For this review, take the finished solid that the model builds, in its own axes (mm). Face numbers are marked on the shaded views. A direction names the side the tool comes from. Coordinates: 2 decimals unless noted, no trailing zeros. Write each loop counter-clockwise with the first axis right and the second up, starting at its lowest first coordinate (ties: lowest second). Pieces come first, ordered by that corner, then holes.
```python
from build123d import *
from OCP.BRepFilletAPI import BRepFilletAPI_MakeChamfer

# Parameters (mm, degrees)
SKETCH1_W           = 96.449496644
SKETCH1_H           = 93.866027984
BOSS_EXTRUDE1_DEPTH = 50
DRAFT1_ANGLE        = 20
CHAMFER1_SIZE       = 5
CHAMFER1_SIZE2      = 8.365785926
CHAMFER2_SIZE       = 2
CHAMFER2_SIZE2      = 3.34631437
SHELL1_T            = -3


with BuildPart() as part:
    # Sketch1 → Boss-Extrude1 (new body)
    with BuildSketch(Plane(origin=(0, 0, 0), x_dir=(1, 0, 0), z_dir=(0, 1, 0))):
        Rectangle(SKETCH1_W, SKETCH1_H)
        Polygon((20.883038336, 70.399520989), (48.224748322, 46.933013992), (-48.224748322, 46.933013992), (-20.883038336, 70.399520989), align=None)
        Polygon((-48.224748322, -46.933013992), (48.224748322, -46.933013992), (20.883038336, -70.399520989), (-20.883038336, -70.399520989), align=None)
    extrude(amount=BOSS_EXTRUDE1_DEPTH)

    # Draft1
    draft1_faces = [part.faces().sort_by_distance(p)[0] for p in [
        (-34.553893329, 25, 58.66626749),
        (-48.224748322, 25, 0),
        (-34.553893329, 25, -58.66626749),
        (0, 25, -70.399520989),
        (34.553893329, 25, -58.66626749),
        (48.224748322, 25, 0),
        (34.553893329, 25, 58.66626749),
        (0, 25, 70.399520989),
    ]]
    draft(draft1_faces, Plane(origin=(0, 0, 0), x_dir=(0, 0, -1), z_dir=(0, -1, 0)), DRAFT1_ANGLE)

    # Chamfer1: one chamfer whose edges measure the first distance from different faces: ONE call of the kernel's chamfer builder (chamfer() names one face for all edges)
    chamfer1_edges_1 = [part.edges().sort_by_distance(p)[0] for p in [
        (0, 0, 70.399520989),
        (-34.553893329, 0, 58.66626749),
        (34.553893329, 0, 58.66626749),
    ]]
    chamfer1_side_1 = [part.faces().sort_by_distance(p)[0] for p in [
        (0, 0, 0),
    ]]
    chamfer1_edges_2 = [part.edges().sort_by_distance(p)[0] for p in [
        (-34.553893329, 0, -58.66626749),
    ]]
    chamfer1_side_2 = [part.faces().sort_by_distance(p)[0] for p in [
        (-41.148260159, 26.443805038, -65.690138569),
    ]]
    chamfer1_edges_3 = [part.edges().sort_by_distance(p)[0] for p in [
        (0, 0, -70.399520989),
    ]]
    chamfer1_side_3 = [part.faces().sort_by_distance(p)[0] for p in [
        (0, 26.157748942, -79.920162999),
    ]]
    chamfer1_edges_4 = [part.edges().sort_by_distance(p)[0] for p in [
        (34.553893329, 0, -58.66626749),
    ]]
    chamfer1_side_4 = [part.faces().sort_by_distance(p)[0] for p in [
        (41.148260159, 26.443805038, -65.690138569),
    ]]
    chamfer1 = BRepFilletAPI_MakeChamfer(part.part.solid().wrapped)
    for e in chamfer1_edges_1:
        chamfer1.Add(CHAMFER1_SIZE, CHAMFER1_SIZE2, e.wrapped, chamfer1_side_1[0].wrapped)  # the first distance lies on this face
    for e in chamfer1_edges_2:
        chamfer1.Add(CHAMFER1_SIZE, CHAMFER1_SIZE2, e.wrapped, chamfer1_side_2[0].wrapped)  # the first distance lies on this face
    for e in chamfer1_edges_3:
        chamfer1.Add(CHAMFER1_SIZE, CHAMFER1_SIZE2, e.wrapped, chamfer1_side_3[0].wrapped)  # the first distance lies on this face
    for e in chamfer1_edges_4:
        chamfer1.Add(CHAMFER1_SIZE, CHAMFER1_SIZE2, e.wrapped, chamfer1_side_4[0].wrapped)  # the first distance lies on this face
    add(Compound.cast(chamfer1.Shape()), mode=Mode.REPLACE)

    # Chamfer2: one chamfer whose edges measure the first distance from different faces: ONE call of the kernel's chamfer builder (chamfer() names one face for all edges)
    chamfer2_edges_1 = [part.edges().sort_by_distance(p)[0] for p in [
        (48.224748322, 0, 2.217733352),
    ]]
    chamfer2_side_1 = [part.faces().sort_by_distance(p)[0] for p in [
        (57.660024046, 25.923206996, -0.008470654),
    ]]
    chamfer2_edges_2 = [part.edges().sort_by_distance(p)[0] for p in [
        (-48.224748322, 0, 2.217733352),
    ]]
    chamfer2_side_2 = [part.faces().sort_by_distance(p)[0] for p in [
        (0, 0, 1.984639343),
    ]]
    chamfer2 = BRepFilletAPI_MakeChamfer(part.part.solid().wrapped)
    for e in chamfer2_edges_1:
        chamfer2.Add(CHAMFER2_SIZE, CHAMFER2_SIZE2, e.wrapped, chamfer2_side_1[0].wrapped)  # the first distance lies on this face
    for e in chamfer2_edges_2:
        chamfer2.Add(CHAMFER2_SIZE, CHAMFER2_SIZE2, e.wrapped, chamfer2_side_2[0].wrapped)  # the first distance lies on this face
    add(Compound.cast(chamfer2.Shape()), mode=Mode.REPLACE)

    # Shell1
    shell1_openings = [part.faces().sort_by_distance(p)[0] for p in [
        (0, 50, 0),
    ]]
    offset(amount=SHELL1_T, openings=shell1_openings, kind=Kind.INTERSECTION)


solid = part.part
```
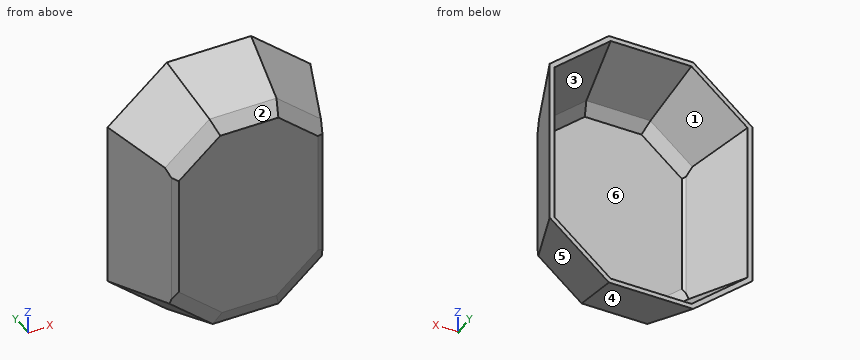
Q1. Add section D-D (y = 24). State the section outline as (x, z) points, then the cut area to 3 significant figures.
Ans:
outline: (-56.96, -50.95) - (-24.12, -79.13) - (24.12, -79.13) - (56.96, -50.95) - (56.96, 50.95) - (24.12, 79.13) - (-24.12, 79.13) - (-56.96, 50.95) - close; hole (-53.77, -49.48) - (-22.94, -75.94) - (22.94, -75.94) - (53.77, -49.48) - (53.77, 49.48) - (22.94, 75.94) - (-22.94, 75.94) - (-53.77, 49.48) - close
area: 1,480 mm2
Q2. Add section B-B (z = 39). State the section outline as (x, y) points, then the cut area to 3 significant figures.
Ans:
outline: (-66.42, 50) - (-49.37, 3.14) - (-46.22, 0) - (44.88, 0) - (48.91, 1.88) - (66.42, 50) - (63.23, 50) - (46.51, 4.07) - (44.21, 3) - (-44.98, 3) - (-46.78, 4.8) - (-63.23, 50) - close
area: 588 mm2
Q3. For probe 1 along Y at (x, z) = (29, 7); probe 2 along X at (y, z) = (44.5, -34); probe 3 along X at (y, z) = (12, 31), list the stretches that pass through material, from the lowest coordinate up.
Ans:
probe 1: y = 0 to 3
probe 2: x = -64.42 to -61.23, 61.23 to 64.42
probe 3: x = -52.59 to -49.4, 49.4 to 52.59
Q4. Tool access review of the marked faces 5 and 6: name each direction out of +Z, -Z, +X, -X, +Y, -Y from which nothing blocks a thin tool from reaching the whole face with its end or side.
Ans:
face 5: -Z, +X, -Y
face 6: +Y
Q5. Add section A-A (y = 16). State the section outline as (x, z) points.
Ans:
outline: (-54.05, -49.61) - (-23.04, -76.22) - (23.04, -76.22) - (54.05, -49.61) - (54.05, 49.61) - (23.04, 76.22) - (-23.04, 76.22) - (-54.05, 49.61) - close; hole (-50.86, -48.14) - (-21.86, -73.03) - (21.86, -73.03) - (50.86, -48.14) - (50.86, 48.14) - (21.86, 73.03) - (-21.86, 73.03) - (-50.86, 48.14) - close
Q6. Clearance check with flat-ended pins moving along their axes: pin 1 Ø10 at (y, z) = (35, 6) entering from +X; pin 2 Ø10 at (x, y) = (-32, 37) entering from +Z; pin 3 Ø12 at (x, y) = (-2, 15) entering from -Z. State where each tip first meets the part, or that it passes through.
Ans:
pin 1: stops at x = 62.78
pin 2: stops at z = 83.52
pin 3: stops at z = -78.04
Q7. Draft analysis for pull direction Z (two halves, no side actions). For the marked faces 1, 2, 3 and 4, state which applies: +Z half, -Z half, draft (parallel to the pull), parting line (faces both ways), or undercut.
Ans:
face 1: undercut
face 2: +Z half
face 3: undercut
face 4: -Z half
Q8. Add section C-C (x = 11.5). State the section outline as (y, z) points, then the cut area to 3 significant figures.
Ans:
outline: (0, -62.03) - (4.7, -72.11) - (50, -88.6) - (50, -85.41) - (6.89, -69.72) - (3, -61.37) - (3, 64.16) - (9.51, 70.67) - (50, 85.41) - (50, 88.6) - (7.86, 73.26) - (0, 65.4) - close
area: 713 mm2
